Can you work these out from the model? Positions are in its coordinate system, mm. A direction names the side the tool comes from. Give positions to 0.01 mm unless a question says otherwise; leave off trailing zeros. Order: outer loops, then holes, each group sorted by start corner. A loop starts at its lowest first (then second) coordinate and runs counter-clockwise, first axis right, second up. Notation, with made-up numbers: M 57,68 L 113,68 A25 cw 113,96 Z; hole C 12.25,52 d2. An arc over 180 degrees is marked long. Use a Markdown table: item, result. Add a question column.
from build123d import *

# Parameters (mm, degrees)
F3_ANGLE = 150
F4_R     = 2.99999
F4_2_R   = 2.99999


# Not quite as in the source:
# - a fillet or chamfer is up to 0.001 mm smaller than in the source, because OpenCascade refuses the exact size


with BuildPart() as f1:
    # F0 (on Front) → F1 (revolve)
    with BuildSketch(Plane.XZ):
        Polygon((-22.5, 0), (-22.5, 30), (-47.5, 30), (-47.5, 20), (-27.5, 0), align=None)
    revolve(axis=Axis((0, 0, 9.4880101401), (0, 0, -1)))


with BuildPart() as f3:
    # F2 (on Front) → F3 (revolve)
    with BuildSketch(Plane.XZ):
        Polygon((-35.2781745931, 14.8492424049), (-39.5208152802, 19.091883092), (-45.1776695297, 13.4350288425), (-40.9350288425, 9.1923881554), align=None)
    revolve(axis=Axis((0, 0, 13.259918429), (0, 0, -1)), revolution_arc=F3_ANGLE)

    # F4 (radius 3 in the source; OpenCascade refuses exactly that, so slightly less here)
    f4_edges = [f3.edges().sort_by_distance(p)[0] for p in [
        (-42.349242, 0, 16.263456),
        (-38.106602, 0, 12.020815),
        (33.001285, 19.053301, 12.020815),
        (36.67552, 21.174621, 16.263456),
    ]]
    fillet(f4_edges, radius=F4_R)


with BuildPart() as f3b:
    # F2 (on Front) → F3, piece 2 (revolve)
    with BuildSketch(Plane.XZ):
        Polygon((-31.7426406871, 11.313708499), (-37.3994949366, 5.6568542495), (-33.1568542495, 1.4142135624), (-27.5, 7.0710678119), align=None)
    revolve(axis=Axis((0, 0, 13.259918429), (0, 0, -1)), revolution_arc=F3_ANGLE)

    # F4#2 (radius 3 in the source; OpenCascade refuses exactly that, so slightly less here)
    f4_2_edges = [f3b.edges().sort_by_distance(p)[0] for p in [
        (-30.328427, 0, 4.242641),
        (-34.571068, 0, 8.485281),
        (26.265188, 15.164214, 4.242641),
        (29.939423, 17.285534, 8.485281),
    ]]
    fillet(f4_2_edges, radius=F4_2_R)


with BuildPart() as f1_1:
    add(f1.part)

    # F5: cut F3b, F3
    add(f3b.part, mode=Mode.SUBTRACT)
    add(f3.part, mode=Mode.SUBTRACT)


solid = f1_1.part
1. Will these pins go through, and if not, where does the flat tip stop? pin 1 (1.8 mm diameter, centred on x = -30.5, z = 7.5, fed in from +Y); pin 2 (3 mm diameter, centred on y = 18.5, z = 18.5, fed in from -X); pin 3 (12 mm diameter, centred on y = -7, z = 10.5, fed in from +X).
2. We'd pull the mould along Z, two halves only. Please class faces 1 (the face through (-10.382, -19.961, 15.21)), 2 (the face through (6.172, -27.794, 0.971)), 3 (the face through (-7.62, 26.6, 6.9)): +Z half, -Z half, draft (parallel to the pull), parting line (faces both ways), or undercut.
3. If we section it at B-B, the plane z = 28: List the corners of the cut face in (x, y) for me.
4. If we section it at A-A, the plane x = 0: List the corners of the cut face in (y, z) for me.
5. I need wall thicknesses on L1, parallel to X at y = 6.5, z = 17; L2, parallel to Y at x = 0, z = 23; L3, parallel to X at y = 6.5, z = 18. Which ranges of each line are inside material? Lowest first, please. Write a range as [from, to].
6. On a 3-axis mill with a long thin cutter (end or side, diameter ignored), from which of +Z, -Z, +X, -X, +Y, -Y can I reach the whole of each face in a straight line? I mean faces 4 (the face through (-9.766, 34.078, 14.678)), 5 (the face through (-7.676, 26.683, 7.336)), 6 (the face through (-8.8, 30.73, 11.09)). Say none if no direction works.
Geometry results:
| question | item | result |
|---|---|---|
| 1 | pin 1 | stops at y = 19.45 |
| 1 | pin 2 | stops at x = -43.87 |
| 1 | pin 3 | stops at x = 43.51 |
| 2 | face 1 | draft |
| 2 | face 2 | -Z half |
| 2 | face 3 | undercut |
| 3 | outline | C 0,0 d95; hole C 0,0 d45 |
| 4 | outline | M -47.5,20 L -27.5,0 L -22.5,0 L -22.5,30 L -47.5,30 Z; M 22.5,0 L 27.5,0 L 31.04,3.54 L 27.5,7.07 L 31.74,11.31 L 35.28,7.78 L 38.81,11.31 L 35.28,14.85 L 39.52,19.09 L 43.06,15.56 L 47.5,20 L 47.5,30 L 22.5,30 Z |
| 5 | L1 | x = [-44.02, -41.1], [-36.86, -21.54], [21.54, 44.02] |
| 5 | L2 | y = [-47.5, -22.5], [22.5, 47.5] |
| 5 | L3 | x = [-45.03, -40.09], [-37.88, -21.54], [21.54, 45.03] |
| 6 | face 4 | +Y |
| 6 | face 5 | none |
| 6 | face 6 | -Z |
